Can you work these out from the model? Positions are in its coordinate system, mm. A direction names the side the tool comes from. Round coordinates to 2 decimals unless told otherwise and drop trailing zeros. Order: outer loops, then holes, each group sorted by start corner. A loop starts at its lowest first (then second) coordinate and runs counter-clockwise, first axis right, second up.
Q1. If I drill on line 1 (Y direction, x = 55, z = 4.05); line 2 (X direction, y = -4.5, z = 1.05); line 3 (X direction, y = 0.75, z = 0.65), over which ranges is the centre line in solid material (lowest first)?
Q2. We'd pull the mould along Y, two halves only. Please class faces 3 (the face through (-5.87, 4.67, 2.46)), 4 (the face through (11.105, -5.719, 1.268)), 5 (the face through (8.7, -1.1, 3.7)), 6 (the face through (26.45, -15.305, 2.465)): pulls with the +Y half, pulls with the -Y half, needs draft (parallel to the pull), parting line crosses it, or undercut.
Q3. If we section it at A-A (z = 1.4): Please give me the cut outline in (x, y) (3 decimals).
Q4. Will these pins go through, and if not, where does the flat tip stop? P1, Ø1.4, axis at x = 10.78, y = -6.22, coming from the +Z side; P2, Ø2.5, axis at x = 55, y = 0, coming from the +Z side.
Q5. If we section it at B-B (x = 0): Please give me the cut outline in (y, z), plus the area to 3 significant figures.
Q6. For faces 1 (the face through (8.608, -4.819, 1.268)), 2 (the face through (8.2, -4.2, 2.5)), which set-ups out of +Z, -Z, +X, -X, +Y, -Y let a thin tool reach every point of the face, with its end or its side?
Q7. If we section it at C-C (y = 0): Please give me the cut outline in (x, z), plus the area to 3 significant figures.
Q8. If we section it at D-D (x = 55): Please give me the cut outline in (y, z), plus the area to 3 significant figures.
from build123d import *

# Parameters (mm, degrees)
SKETCH1_R           = 7.5
SKETCH1_R_2         = 5
SKETCH1_R_3         = 2.5
SKETCH1_R_4         = 1.5
BOSS_EXTRUDE1_DEPTH = 5
SKETCH2_R           = 0.6
CUT_EXTRUDE1_DEPTH  = 10
CUT_EXTRUDE2_START  = -2.5
CUT_EXTRUDE2_DEPTH  = 2.5


with BuildPart() as part:
    # Sketch1 → Boss-Extrude1 (new body)
    # profile 1 of 3: a face of its own
    with BuildSketch(Plane.XY):
        with BuildLine():
            ThreePointArc((53.791866029, 2.188701055), (28.624593116, -3.284466085), (4.577922078, 5.940760006))
            ThreePointArc((4.577922078, 5.940760006), (6.729948573, 3.310255611), (7.5, 0))
            ThreePointArc((7.5, 0), (3.356031274, -6.707238932), (-4.496547756, -6.002587632))
            ThreePointArc((-4.496547756, -6.002587632), (26.917032253, -15.274892681), (56.759448417, -1.776046528))
            ThreePointArc((56.759448417, -1.776046528), (52.998552336, -1.498067838), (53.791866029, 2.188701055))
        make_face()
    # profile 2 of 3: a face of its own
    with BuildSketch(Plane.XY):
        Circle(SKETCH1_R)
        Circle(SKETCH1_R_2, mode=Mode.SUBTRACT)
    # profile 3 of 3: a face of its own
    with BuildSketch(Plane.XY):
        with Locations((55, 0)):
            Circle(SKETCH1_R_3)
        with Locations((55, 0)):
            Circle(SKETCH1_R_4, mode=Mode.SUBTRACT)
    extrude(amount=BOSS_EXTRUDE1_DEPTH)

    # Sketch2 → Cut-Extrude1 (cut)
    with BuildSketch(Plane.XY.offset(5)):
        with Locations((3.853813047, -2.225)):
            Circle(SKETCH2_R)
        with Locations((5.585863854, -3.225)):
            Circle(SKETCH2_R)
        with Locations((7.317914662, -4.225)):
            Circle(SKETCH2_R)
        with Locations((9.04996547, -5.225)):
            Circle(SKETCH2_R)
        with Locations((10.782016277, -6.225)):
            Circle(SKETCH2_R)
        with Locations((12.514067085, -7.225)):
            Circle(SKETCH2_R)
    extrude(amount=-CUT_EXTRUDE1_DEPTH, mode=Mode.SUBTRACT)

    # Sketch3 → Cut-Extrude2 (cut)
    with BuildSketch(Plane.XY.offset(5).offset(CUT_EXTRUDE2_START)):
        with BuildLine():
            Line((13.851873565, -5.738301032), (3.344516201, 3.71674742))
            ThreePointArc((3.344516201, 3.71674742), (4.330127019, -2.5), (-1.546539584, -4.754809703))
            Line((-1.546539584, -4.754809703), (11.895451251, -9.126923881))
            ThreePointArc((11.895451251, -9.126923881), (14.246117892, -8.225), (13.851873565, -5.738301032))
        make_face()
    extrude(amount=CUT_EXTRUDE2_DEPTH, mode=Mode.SUBTRACT)


solid = part.part
Solution:
1. line 1: y = -3.43 to -1.5, 1.5 to 2.5
1. line 2: x = -6 to -2.18, 2.18 to 6.78, 7.85 to 53.76
1. line 3: x = -7.46 to -4.94, 4.94 to 13.14, 50.95 to 53.7, 56.3 to 57.38
2. face 3: parting line crosses it
2. face 4: undercut
2. face 5: undercut
2. face 6: pulls with the -Y half
3. outline: (-4.497, -6.003) arc R47 ccw to (56.759, -1.776) arc R2.5 ccw to (53.792, 2.189) arc R45 cw to (4.578, 5.941) arc R7.5 ccw (long way) to start; hole (4.197, -2.717) arc R0.6 ccw to (4.452, -2.277) arc R5 ccw (long way) to start; hole circle Ø1.2 at (5.586, -3.225); hole circle Ø1.2 at (7.318, -4.225); hole circle Ø1.2 at (9.05, -5.225); hole circle Ø1.2 at (10.782, -6.225); hole circle Ø1.2 at (12.514, -7.225); hole circle Ø3 at (55, 0)
4. P1: stops at z = 2.5
4. P2: passes through
5. outline: (-8.98, 0) - (-5, 0) - (-5, 2.5) - (-5.26, 2.5) - (-5.26, 5) - (-8.98, 5) - close; (5, 0) - (7.5, 0) - (7.5, 5) - (5, 5) - close
5. area: 31.8 mm2
6. face 1: +Z, -Z
6. face 2: +Z
7. outline: (-7.5, 0) - (-5, 0) - (-5, 5) - (-7.5, 5) - close; (5, 0) - (14.85, 0) - (14.85, 5) - (7.47, 5) - (7.47, 2.5) - (5, 2.5) - close; (49.24, 0) - (53.5, 0) - (53.5, 5) - (49.24, 5) - close; (56.5, 0) - (57.5, 0) - (57.5, 5) - (56.5, 5) - close
7. area: 81.9 mm2
8. outline: (-3.43, 0) - (-1.5, 0) - (-1.5, 5) - (-3.43, 5) - close; (1.5, 0) - (2.5, 0) - (2.5, 5) - (1.5, 5) - close
8. area: 14.7 mm2
